Can you work these out from the model? Positions are in its coordinate system, mm. A direction names the side the tool comes from. Coordinates: 2 decimals unless noted, no trailing zeros. Loops run counter-clockwise (first coordinate to the right, second up) from the corner with the lowest first, then second, coordinate; pieces in that order, holes last. Notation, with made-up numbers: (-18, 19.5) -> (13, 19.5) arc R26 cw to (13, 34.5) -> close; hole circle Ø9 at (-31, 88). An arc over 180 degrees is marked (long way). Use one line per item in the form item = value. Start each with the question number.
(1) Imagine slicing it at B-B (y = -20). List the corners of the cut face in (x, z) for me.
(2) I need wall thicknesses on line 1 (Y direction, x = -19.85, z = 0.75); line 2 (Y direction, x = 4, z = 0.35); line 3 (Y direction, x = 0, z = 2.1). Which ranges of each line are inside material? Lowest first, please. Write a range as [from, to].
(3) Imagine slicing it at A-A (x = 19.85). List the corners of the cut face in (y, z) for me.
(4) Imagine slicing it at C-C (z = 0.65). State how many separate pieces and enclosed holes the cut face has, plus the area to 3 significant figures.
(5) Imagine slicing it at D-D (x = 11). List the corners of the cut face in (y, z) for me.
(6) Thinking about a two-plate mould opening in X: for faces 1 (the cylindrical face through (31.89, 31.85, 1.48)), 2 (the flat face through (0, -17.5, 1)), 3 (the cylindrical face through (-31.85, 31.89, 1.48)), which applies, released by +X, released by -X, zero draft, split by the parting line, or undercut?
(7) On a 3-axis mill with a long thin cutter (end or side, diameter ignored), from which of +Z, -Z, +X, -X, +Y, -Y can I reach the whole of each face in a straight line? I mean faces 4 (the flat face through (0, -32.75, 1)), 5 (the cylindrical face through (-12.5, -19.9, 1.5)). Say none if no direction works.
```python
from build123d import *

# Parameters (mm, degrees)
SKETCH_R   = 2.55
SKETCH_R_2 = 3.6
PAD_DEPTH  = 3


with BuildPart() as part:
    # Sketch → Pad (new body)
    with BuildSketch(Plane.XY):
        with BuildLine():
            ThreePointArc((-29.75, 32.75), (-31.87132, 31.87132), (-32.75, 29.75))
            Line((-32.75, -29.75), (-32.75, 29.75))
            ThreePointArc((-32.75, -29.75), (-31.87132, -31.87132), (-29.75, -32.75))
            Line((29.75, -32.75), (-29.75, -32.75))
            ThreePointArc((29.75, -32.75), (31.87132, -31.87132), (32.75, -29.75))
            Line((32.75, 29.75), (32.75, -29.75))
            ThreePointArc((32.75, 29.75), (31.87132, 31.87132), (29.75, 32.75))
            Line((-29.75, 32.75), (29.75, 32.75))
        make_face()
        Circle(SKETCH_R, mode=Mode.SUBTRACT)
        with Locations((-19.85, -20)):
            Circle(SKETCH_R_2, mode=Mode.SUBTRACT)
        with Locations((19.85, -20)):
            Circle(SKETCH_R_2, mode=Mode.SUBTRACT)
        with Locations((19.85, 20)):
            Circle(SKETCH_R_2, mode=Mode.SUBTRACT)
        with Locations((-19.85, 20)):
            Circle(SKETCH_R_2, mode=Mode.SUBTRACT)
        with Locations((-19.85, 0)):
            Circle(SKETCH_R, mode=Mode.SUBTRACT)
        with Locations((19.85, 0)):
            Circle(SKETCH_R_2, mode=Mode.SUBTRACT)
        with BuildLine():
            ThreePointArc((-10, -17.5), (-12.5, -20), (-10, -22.5))
            Line((-10, -22.5), (10, -22.5))
            ThreePointArc((10, -22.5), (12.5, -20), (10, -17.5))
            Line((10, -17.5), (-10, -17.5))
        make_face(mode=Mode.SUBTRACT)
        with BuildLine():
            ThreePointArc((-10, 22.5), (-12.5, 20), (-10, 17.5))
            Line((-10, 17.5), (10, 17.5))
            ThreePointArc((10, 17.5), (12.5, 20), (10, 22.5))
            Line((10, 22.5), (-10, 22.5))
        make_face(mode=Mode.SUBTRACT)
    extrude(amount=PAD_DEPTH)


solid = part.part
```
Worked out:
q1.outline = (-32.75, 0) -> (-23.45, 0) -> (-23.45, 3) -> (-32.75, 3) -> close; (-16.25, 0) -> (-12.5, 0) -> (-12.5, 3) -> (-16.25, 3) -> close; (12.5, 0) -> (16.25, 0) -> (16.25, 3) -> (12.5, 3) -> close; (23.45, 0) -> (32.75, 0) -> (32.75, 3) -> (23.45, 3) -> close
q2.line_1 = [-32.75, -23.6], [-16.4, -2.55], [2.55, 16.4], [23.6, 32.75]
q2.line_2 = [-32.75, -22.5], [-17.5, 17.5], [22.5, 32.75]
q2.line_3 = [-32.75, -22.5], [-17.5, -2.55], [2.55, 17.5], [22.5, 32.75]
q3.outline = (-32.75, 0) -> (-23.6, 0) -> (-23.6, 3) -> (-32.75, 3) -> close; (-16.4, 0) -> (-3.6, 0) -> (-3.6, 3) -> (-16.4, 3) -> close; (3.6, 0) -> (16.4, 0) -> (16.4, 3) -> (3.6, 3) -> close; (23.6, 0) -> (32.75, 0) -> (32.75, 3) -> (23.6, 3) -> close
q4.separate_pieces = 1
q4.enclosed_holes = 9
q4.area = 3,800 mm2
q5.outline = (-32.75, 0) -> (-22.29, 0) -> (-22.29, 3) -> (-32.75, 3) -> close; (-17.71, 0) -> (17.71, 0) -> (17.71, 3) -> (-17.71, 3) -> close; (22.29, 0) -> (32.75, 0) -> (32.75, 3) -> (22.29, 3) -> close
q6.face_1 = released by +X
q6.face_2 = undercut
q6.face_3 = released by -X
q7.face_4 = +Z, -Z, +X, -X, -Y
q7.face_5 = +Z, -Z
